Part model, mm, in its own coordinate system. Round coordinates to 2 decimals unless told otherwise and drop trailing zeros. Write each loop counter-clockwise with the first axis right and the second up, starting at its lowest first coordinate (ties: lowest second). Pieces come first, ordered by that corner, then holes. Notation, with made-up numbers: (55.5, -12.75) -> (105.5, -12.75) arc R24 cw to (105.5, 23.25) -> close; hole circle Ø3 at (-26.75, 61). An arc over 180 degrees is marked (long way). Use CSV: the item, a comma, the result in double quotes. Start each with the question number.
Autodesk Inventor part; units mm, degrees
ref_plane "YZ Plane" through (0, 0, 0) normal (1, 0, 0) x (0, 1, 0)
ref_plane "XZ Plane" through (0, 0, 0) normal (0, 1, 0) x (-1, 0, 0)
ref_plane "XY Plane" through (0, 0, 0) normal (0, 0, 1) x (1, 0, 0)
sketch "Sketch1" plane through (0, 0, 0) normal (0, 1, 0) x (-1, 0, 0)
  circle A0 centre (0, 0) radius 30
  circle A1 centre (0, 0) radius 26
  dimension "d0" = 60
  dimension "d1" = 52
extrude "Extrusion1" add sketch "Sketch1" along normal blind 3.5
sketch "Sketch2" plane through (0, 3.5, 0) normal (0, 1, 0) x (1, 0, 0)
  circle A0 centre (0, 0) radius 1.25
  line L0 (0, -27.5) -> (0, 0) construction
  circle A1 centre (0, 0) radius 60 construction
  line L1 (-1.9903, -27.4279) -> (-3.0861, -9.5119)
  line L2 (1.9903, -27.4279) -> (3.0861, -9.5119)
  arc A2 (-0.5773, -24.0366) -> (0.6206, -24.0343) centre (0.0216, -24) ccw
  arc A3 (1.248, -13.0714) -> (-1.2477, -13.0763) centre (0, -13) ccw
  line L3 (-1.2477, -13.0763) -> (-0.5773, -24.0366)
  line L4 (0.6206, -24.0343) -> (1.248, -13.0714)
  line L5 (-2.2, -24) -> (2.2, -24) construction
  line L6 (25.4704, -10.3686) -> (8.0927, -5.8744)
  line L7 (26.7005, -6.5828) -> (10, -0.0042)
  line L8 (23.0497, -6.8368) -> (12.8173, -2.8524)
  arc A4 (12.8173, -2.8524) -> (12.0508, -5.2274) centre (12.3637, -4.0172) ccw
  line L9 (12.0508, -5.2274) -> (22.6818, -7.9768)
  arc A5 (22.6818, -7.9768) -> (23.0497, -6.8368) centre (22.832, -7.3959) ccw
  line L10 (17.7319, 21.0197) -> (8.0877, 5.8813)
  line L11 (14.5115, 23.3595) -> (3.0942, 9.5093)
  line L12 (13.6249, 19.8089) -> (6.6736, 11.3085)
  arc A6 (6.6736, 11.3085) -> (8.6954, 9.8456) centre (7.6412, 10.5172) ccw
  line L13 (8.6954, 9.8456) -> (14.5954, 19.1067)
  arc A7 (14.5954, 19.1067) -> (13.6249, 19.8089) centre (14.0894, 19.4291) ccw
  line L14 (-14.5115, 23.3595) -> (-3.0942, 9.5093)
  line L15 (-17.7319, 21.0197) -> (-8.0877, 5.8813)
  line L16 (-14.6291, 19.0794) -> (-8.6928, 9.8415)
  arc A8 (-8.6928, 9.8415) -> (-6.6767, 11.3123) centre (-7.6412, 10.5172) ccw
  line L17 (-6.6767, 11.3123) -> (-13.6613, 19.7854)
  arc A9 (-13.6613, 19.7854) -> (-14.6291, 19.0794) centre (-14.1243, 19.4037) ccw
  line L18 (-26.7005, -6.5828) -> (-10, -0.0042)
  line L19 (-25.4704, -10.3686) -> (-8.0927, -5.8744)
  line L20 (-22.6662, -8.0172) -> (-12.046, -5.2262)
  arc A10 (-12.046, -5.2262) -> (-12.8219, -2.8542) centre (-12.3637, -4.0172) ccw
  line L21 (-12.8219, -2.8542) -> (-23.0386, -6.8787)
  arc A11 (-23.0386, -6.8787) -> (-22.6662, -8.0172) centre (-22.8187, -7.4369) ccw
  arc A12 (-1.9903, -27.4279) -> (1.9903, -27.4279) centre (0, 0) ccw
  arc A13 (25.4704, -10.3686) -> (26.7005, -6.5828) centre (0, 0) ccw
  arc A14 (17.7319, 21.0197) -> (14.5115, 23.3595) centre (0, 0) ccw
  arc A15 (-14.5115, 23.3595) -> (-17.7319, 21.0197) centre (0, 0) ccw
  arc A16 (-26.7005, -6.5828) -> (-25.4704, -10.3686) centre (0, 0) ccw
  arc A17 (3.0861, -9.5119) -> (8.0927, -5.8744) centre (0, 0) ccw
  arc A18 (10, -0.0042) -> (8.0877, 5.8813) centre (0, 0) ccw
  arc A19 (3.0942, 9.5093) -> (-3.0942, 9.5093) centre (0, 0) ccw
  arc A20 (-8.0877, 5.8813) -> (-10, -0.0042) centre (0, 0) ccw
  arc A21 (-8.0927, -5.8744) -> (-3.0861, -9.5119) centre (0, 0) ccw
  circle A22 centre (0, 0) radius 6.25 construction
  circle A23 centre (0, 6.25) radius 1.5
  circle A24 centre (0, -6.25) radius 1.5
  point P0 (22.1455, -9.5087)
  point P1 (23.5052, -5.3241)
  point P2 (15.8867, 18.1233)
  point P3 (12.327, 20.7095)
  point P4 (-12.327, 20.7095)
  point P5 (-15.8867, 18.1233)
  point P6 (-23.5052, -5.3241)
  point P7 (-22.1455, -9.5087)
  dimension "d11" = 2.5
  dimension "d13" = 120
  dimension "d15" = 3.5
  dimension "d17" = 0.6
  dimension "d18" = 2.5
  dimension "d19" = 24
  dimension "d20" = 13
  dimension "d21" = 0.225
  dimension "d22" = 4.4
  dimension "d25" = 360
  dimension "d27" = 10
  dimension "d28" = 27.5
  dimension "d29" = 12.5
  dimension "d30" = 3
extrude "Extrusion2" add sketch "Sketch2" against normal up to surface (3.5 mm away)
properties part number "wheel"
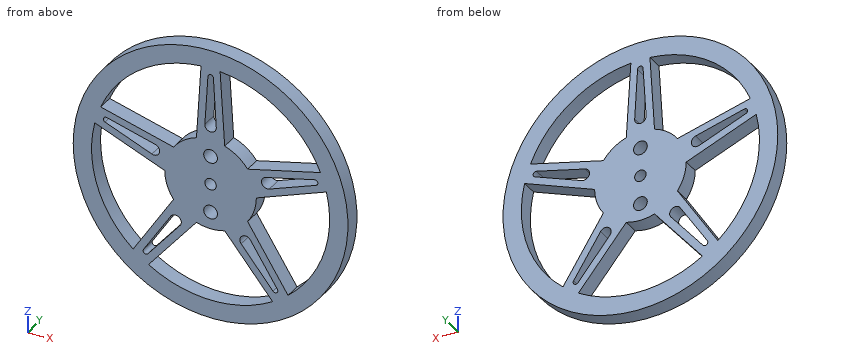
1. Drill centre lines: line 1 along Z through (x, y) = (0, 2.35); line 2 along X through (y, z) = (1.5, 23); line 3 along X through (y, z) = (1.7, -17). Where is each one in solid material? Low to high. Write a range as [from, to].
2. Band-saw the part on D-D (y = 0.7). Give the number of separate pieces and of enclosed holes in the cut face, then the cut area to 3 significant figures.
3. Band-saw the part on C-C (x = 4). List the corners of the cut face in (y, z).
4. Flat gauge pin, fed straight in: pin 1 (1.5 mm diameter, centred on x = 17, y = 1.5, fed in from -Z). Where does the tip first touch, or does it go through?
5. Band-saw the part on A-A (x = -21.5). List the corners of the cut face in (y, z), then the cut area to 3 significant figures.
6. Band-saw the part on B-B (z = -16). List the corners of the cut face in (x, y), then the cut area to 3 significant figures.
Answers below:
1,line 1,"z = [-30, -26], [-10, -7.75], [-4.75, -1.25], [1.25, 4.75], [7.75, 11.75], [24.6, 30]"
1,line 2,"x = [-19.26, -12.12], [-2.26, -0.64], [0.68, 2.26], [12.12, 19.26]"
1,line 3,"x = [-24.72, -19.67], [-15.17, -13.29], [-11.37, -9.27], [9.27, 11.33], [13.25, 15.17], [19.67, 24.72]"
2,separate pieces,"1"
2,enclosed holes,"13"
2,area,"1,300 mm^2"
3,outline,"(0, -29.73) -> (3.5, -29.73) -> (3.5, -25.69) -> (0, -25.69) -> close; (0, -10.61) -> (3.5, -10.61) -> (3.5, 9.17) -> (0, 9.17) -> close; (0, 25.69) -> (3.5, 25.69) -> (3.5, 29.73) -> (0, 29.73) -> close"
4,pin 1,"stops at z = -25.22"
5,outline,"(0, -20.92) -> (3.5, -20.92) -> (3.5, -14.62) -> (0, -14.62) -> close; (0, 4.53) -> (3.5, 4.53) -> (3.5, 6.27) -> (0, 6.27) -> close; (0, 7.71) -> (3.5, 7.71) -> (3.5, 9.34) -> (0, 9.34) -> close; (0, 14.62) -> (3.5, 14.62) -> (3.5, 20.92) -> (0, 20.92) -> close"
5,area,"55.9 mm^2"
6,outline,"(-25.38, 0) -> (-20.49, 0) -> (-20.49, 3.5) -> (-25.38, 3.5) -> close; (-14.53, 0) -> (-12.65, 0) -> (-12.65, 3.5) -> (-14.53, 3.5) -> close; (-10.54, 0) -> (-8.44, 0) -> (-8.44, 3.5) -> (-10.54, 3.5) -> close; (8.44, 0) -> (10.51, 0) -> (10.51, 3.5) -> (8.44, 3.5) -> close; (12.62, 0) -> (14.53, 0) -> (14.53, 3.5) -> (12.62, 3.5) -> close; (20.49, 0) -> (25.38, 0) -> (25.38, 3.5) -> (20.49, 3.5) -> close"
6,area,"62.1 mm^2"
